Drawing for the job (mm, zero at the part's lowest x, y, z). Coordinates: 2 decimals unless noted, no trailing zeros. Write each loop counter-clockwise with the first axis right and the second up, starting at its lowest first coordinate (ties: lowest second). Pieces come first, ordered by that corner, then holes. Notation, with made-up numbers: (-26, 11) -> (21, 11) arc R15 cw to (21, 20) -> close; hole circle Ø5 at (-29.75, 77). An arc over 180 degrees is marked (long way). Answer as CSV lines item,"result". Start each with the question number.
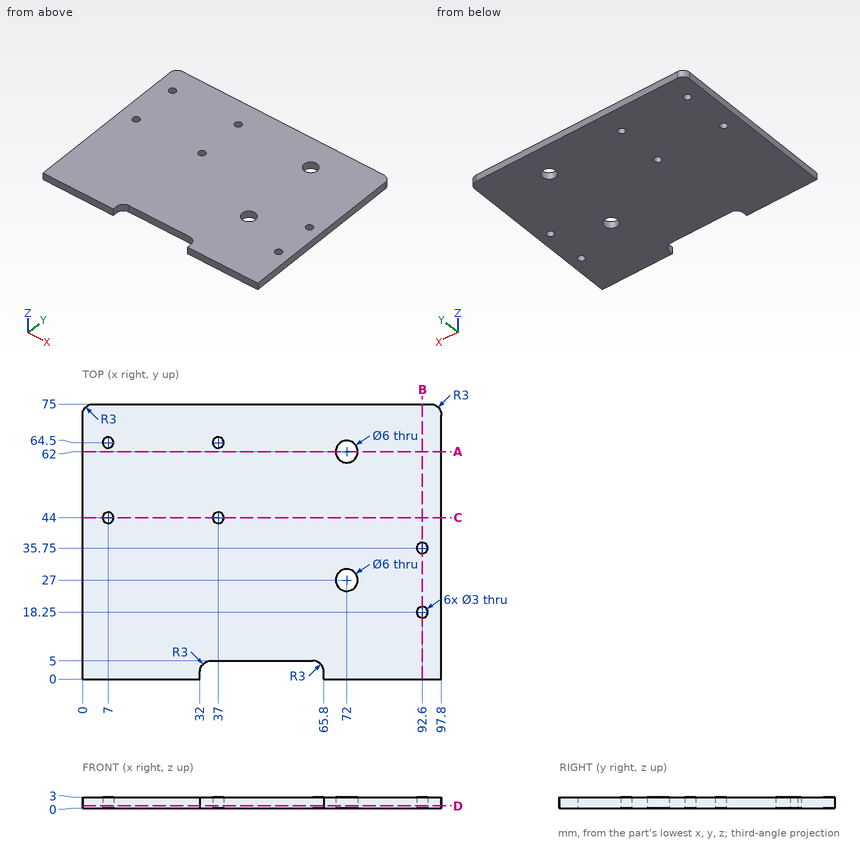
1. Cut at B-B (x = 92.6). Give the cut face in (y, z).
2. Flat gauge pin, fed straight in: P1, Ø1.5, axis at x = 48, z = 2, coming from the -Y side. Where does the tip first touch, or does it go through?
3. Cut at C-C (y = 44). Give the cut face in (x, z), then the cut area to 3 significant figures.
4. Wall check: line 1 (Y direction, x = 72, z = 0.7); line 2 (Y direction, x = 7, z = 0.3); line 3 (Y direction, x = 63, z = 2). Give the ranges that are in metal, low to high.
5. Cut at D-D (z = 0.6). Count the separate pieces of the cut face and the enclosed holes in it, then the cut area to 3 significant figures.
6. Cut at A-A (y = 62). Give the cut face in (x, z).
Geometry check:
1,outline,"(0, 0) -> (16.75, 0) -> (16.75, 3) -> (0, 3) -> close; (19.75, 0) -> (34.25, 0) -> (34.25, 3) -> (19.75, 3) -> close; (37.25, 0) -> (75, 0) -> (75, 3) -> (37.25, 3) -> close"
2,P1,"y = 5"
3,outline,"(0, 0) -> (5.5, 0) -> (5.5, 3) -> (0, 3) -> close; (8.5, 0) -> (35.5, 0) -> (35.5, 3) -> (8.5, 3) -> close; (38.5, 0) -> (97.8, 0) -> (97.8, 3) -> (38.5, 3) -> close"
3,area,"275 mm²"
4,line 1,"0 to 24, 30 to 59, 65 to 75"
4,line 2,"0 to 42.5, 45.5 to 63, 66 to 75"
4,line 3,"4.99 to 75"
5,separate pieces,"1"
5,enclosed holes,"8"
5,area,"7,070 mm²"
6,outline,"(0, 0) -> (69, 0) -> (69, 3) -> (0, 3) -> close; (75, 0) -> (97.8, 0) -> (97.8, 3) -> (75, 3) -> close"
